```python
from build123d import *

# Parameters (mm, degrees)
SKETCH_1_W          = 10
SKETCH_1_H          = 10
SKETCH_1_W_2        = 8
SKETCH_1_H_2        = 8
EXTRUDE_1_DEPTH     = 230
SKETCH_2_R          = 2.15
CUT_EXTRUDE_1_DEPTH = 231.271578793
SKETCH_3_R          = 2.15
CUT_EXTRUDE_2_DEPTH = 231.271578793


with BuildPart() as part:
    # ｽｹｯﾁ1 → 押し出し-薄板1 (new body)
    with BuildSketch(Plane(origin=(0, 0, 0), x_dir=(1, 0, 0), z_dir=(0, 1, 0))):
        Rectangle(SKETCH_1_W, SKETCH_1_H)
        Rectangle(SKETCH_1_W_2, SKETCH_1_H_2, mode=Mode.SUBTRACT)
    extrude(amount=EXTRUDE_1_DEPTH)

    # ｽｹｯﾁ2 → ｶｯﾄ - 押し出し1 (cut, through all)
    with BuildSketch(Plane(origin=(0, 0, 5), x_dir=(-1, 0, 0), z_dir=(0, 0, -1))):
        with Locations((0, 215)):
            Circle(SKETCH_2_R)
        with Locations((0, 225)):
            Circle(SKETCH_2_R)
    extrude(amount=CUT_EXTRUDE_1_DEPTH, mode=Mode.SUBTRACT)

    # ｽｹｯﾁ3 → ｶｯﾄ - 押し出し2 (cut, through all)
    with BuildSketch(Plane(origin=(5, 0, 0), x_dir=(0, 0, -1), z_dir=(1, 0, 0))):
        with Locations((0, 15)):
            Circle(SKETCH_3_R)
        with Locations((0, 5)):
            Circle(SKETCH_3_R)
    extrude(amount=-CUT_EXTRUDE_2_DEPTH, mode=Mode.SUBTRACT)


solid = part.part
```
Source: CAD feature listing. Evaluate the final solid. Frame: model axes, mm. A direction names the side the tool comes from. Round coordinates to 2 decimals unless told otherwise and drop trailing zeros. Loops run counter-clockwise (first coordinate to the right, second up) from the corner with the lowest first, then second, coordinate; pieces in that order, holes last. Notation, with made-up numbers: M 3.5,71.5 L 47.5,71.5 A5 ccw 47.5,80.5 Z; hole C 78,55 d11. An arc over 180 degrees is marked long. Use a Markdown table: item, result. Add a question column.
1. Section query A-A on x = 0. Return the cut outline in (y, z).
2. Section query B-B on y = 215. Return the cut outline in (x, z), then the cut area to 3 significant figures.
3. Section query C-C on z = 0. Return the cut outline in (x, y).
4. Section query D-D on y = 24. Return the cut outline in (x, z), then the cut area to 3 significant figures.
5. Line query: line 1 (Y direction, x = 0, z = -4.45); line 2 (Y direction, x = -4.3, z = 0); line 3 (X direction, y = 175, z = -1.5). Output: solid intervals per line, ascending.
6. Mould query, pull axis Y, two halves, no side actions, for faces 3 (the flat face through (-4.5, 230, -0.1)), 4 (the cylindrical face through (-4.49, 12.9, 0.47)), 5 (the flat face through (-5, 113, 0)). Classes: pulls with the +Y half, pulls with the -Y half, needs draft (parallel to the pull), parting line crosses it, or undercut.
7. Reachability of faces 1 (the flat face through (5, 113, 0)), 2 (the flat face through (0, 113, -4)) from +Z, -Z, +X, -X, +Y, -Y: full face, straight path, thin tool, end or side. Return the list, or none.
Reported:
| question | item | result |
|---|---|---|
| 1 | outline | M 0,-5 L 212.85,-5 L 212.85,-4 L 0,-4 Z; M 0,4 L 212.85,4 L 212.85,5 L 0,5 Z; M 217.15,-5 L 222.85,-5 L 222.85,-4 L 217.15,-4 Z; M 217.15,4 L 222.85,4 L 222.85,5 L 217.15,5 Z; M 227.15,-5 L 230,-5 L 230,-4 L 227.15,-4 Z; M 227.15,4 L 230,4 L 230,5 L 227.15,5 Z |
| 2 | outline | M -5,-5 L -2.15,-5 L -2.15,-4 L -4,-4 L -4,4 L -2.15,4 L -2.15,5 L -5,5 Z; M 2.15,-5 L 5,-5 L 5,5 L 2.15,5 L 2.15,4 L 4,4 L 4,-4 L 2.15,-4 Z |
| 2 | area | 27.4 mm² |
| 3 | outline | M -5,0 L -4,0 L -4,2.85 L -5,2.85 Z; M -5,7.15 L -4,7.15 L -4,12.85 L -5,12.85 Z; M -5,17.15 L -4,17.15 L -4,230 L -5,230 Z; M 4,0 L 5,0 L 5,2.85 L 4,2.85 Z; M 4,7.15 L 5,7.15 L 5,12.85 L 4,12.85 Z; M 4,17.15 L 5,17.15 L 5,230 L 4,230 Z |
| 4 | outline | M -5,-5 L 5,-5 L 5,5 L -5,5 Z; hole M -4,-4 L 4,-4 L 4,4 L -4,4 Z |
| 4 | area | 36.0 mm² |
| 5 | line 1 | y = 0 to 212.85, 217.15 to 222.85, 227.15 to 230 |
| 5 | line 2 | y = 0 to 2.85, 7.15 to 12.85, 17.15 to 230 |
| 5 | line 3 | x = -5 to -4, 4 to 5 |
| 6 | face 3 | pulls with the +Y half |
| 6 | face 4 | undercut |
| 6 | face 5 | needs draft |
| 7 | face 1 | +Z, -Z, +X, +Y, -Y |
| 7 | face 2 | +Y, -Y |
